Read the model definition and answer for the solid it produces. Units are mm, in the model's axes. A direction names the side the tool comes from. Give positions to 0.01 mm unless a question says otherwise; leave off trailing zeros. Write each loop counter-clockwise with the first axis right and the second up, starting at its lowest first coordinate (ties: lowest second). Pieces come first, ordered by that corner, then holes. Notation, with made-up numbers: (35.25, 58.5) -> (57.25, 58.5) arc R18 cw to (57.25, 63.5) -> close; hole circle Ø1 at (-11, 17.25). An arc over 180 degrees is marked (long way). Answer as CSV lines item,"result". Start each with the question number.
1. The part is cut by section C-C, the plane y = -49. Determine the outline of the cut face in (x, z) (1 decimal), and give its area (3 significant figures).
2. Given pin 1 (1.4 mm diameter, centred on y = -80.5, z = -0.5, fed in from -X); pin 2 (3 mm diameter, centred on y = -49.5, z = -6.5, fed in from -X); pin 3 (2 mm diameter, centred on y = -49.5, z = 1, fed in from +X), each flat-ended and moving along its own axis, determine where each tip first touches the part or whether it passes through.
3. The part is cut by section B-B, the plane y = -60. Determine the outline of the cut face in (x, z).
4. Find the intervals of material crossed by line 1 (Y direction, x = -90.5, z = 5.5); line 2 (X direction, y = -78, z = -5.5); line 3 (X direction, y = -75, z = 3.25), in increasing order.
5. The part is cut by section A-A, the plane x = -37. Determine the outline of the cut face in (y, z), and give its area (3 significant figures).
6. The part is cut by section D-D, the plane x = -15. Determine the outline of the cut face in (y, z), and give its area (3 significant figures).
7. A tool of negligible diameter and unlimited length cuts with its end or side. For faces 1 (the flat face through (-102.743, -74, -3)), 2 (the cylindrical face through (-22.46, -91.86, -1.69)), 3 (the cylindrical face through (-7.404, -76.068, -2.685)), 4 (the cylindrical face through (-22.46, -47.07, -1.69)), from which of +Z, -Z, +X, -X, +Y, -Y can it reach the whole face along a straight path? Write none if from no direction.
8. For a pull along Y with two mould halves and no side action, classify faces 5 (the cylindrical face through (-112.375, -77.345, 0.151)), 6 (the flat face through (-109.22, -80, 0)), 7 (the flat face through (-20, -50.165, 0)), 8 (the cylindrical face through (-93.667, -47.074, 0.909)) as pulls with the +Y half, pulls with the -Y half, needs draft (parallel to the pull), parting line crosses it, or undercut.
from build123d import *

# Parameters (mm, degrees)
SKETCH002_W     = 82.55
SKETCH002_H     = 25.4
PAD001_DEPTH    = 19.05
SKETCH003_R     = 5.08
POCKET001_DEPTH = 114.301
SKETCH100_R     = 2.286
POCKET027_DEPTH = 6.223
SKETCH101_R     = 7.14375
POCKET028_DEPTH = 12.7
SKETCH118_R     = 2.8575
POCKET042_DEPTH = 6.096


with BuildPart() as part:
    # Sketch002 → Pad001 (new body)
    with BuildSketch(Plane.XY):
        Polygon((-57.15, 14.589816), (-57.15, -14.589816), (-46.339816, -25.4), (46.339816, -25.4), (57.15, -14.589816), (57.15, 14.589816), (46.339816, 25.4), (-46.339816, 25.4), align=None)
        Rectangle(SKETCH002_W, SKETCH002_H, mode=Mode.SUBTRACT)
    extrude(amount=PAD001_DEPTH)

    # Sketch003 (on Face1 of Pad001) → Pocket001 (cut, through all)
    with BuildSketch(Plane(origin=(-57.15, 0, 0), x_dir=(0, -1, 0), z_dir=(-1, 0, 0))):
        with Locations((0, 9.525)):
            Circle(SKETCH003_R)
    extrude(amount=-POCKET001_DEPTH, mode=Mode.SUBTRACT)

    # Sketch100 (on Face1 of Pocket001) → Pocket027 (cut)
    with BuildSketch(Plane(origin=(-57.15, 0, 0), x_dir=(0, -1, 0), z_dir=(-1, 0, 0))):
        with Locations((10.16, 9.525)):
            Circle(SKETCH100_R)
        with Locations((-10.16, 9.525)):
            Circle(SKETCH100_R)
    extrude(amount=-POCKET027_DEPTH, mode=Mode.SUBTRACT)

    # Sketch101 (on Face1 of Pocket027) → Pocket028 (cut)
    with BuildSketch(Plane(origin=(-57.15, 0, 0), x_dir=(0, -1, 0), z_dir=(-1, 0, 0))):
        with Locations((0, 9.525)):
            Circle(SKETCH101_R)
    pocket028 = extrude(amount=-POCKET028_DEPTH, mode=Mode.SUBTRACT)

    # Mirrored002: Pocket028 across YZ
    add(pocket028.mirror(Plane.YZ), mode=Mode.SUBTRACT)

    # Sketch118 (on Face10 of Mirrored002) → Pocket042 (cut)
    with BuildSketch(Plane.XZ.offset(25.4)):
        with Locations((0, 9.525)):
            Circle(SKETCH118_R)
        with Locations((38.1, 9.525)):
            Circle(SKETCH118_R)
        with Locations((-38.1, 9.525)):
            Circle(SKETCH118_R)
    pocket042 = extrude(amount=-POCKET042_DEPTH, mode=Mode.SUBTRACT)

    # Mirrored004: Pocket042 across XZ
    add(pocket042.mirror(Plane.XZ), mode=Mode.SUBTRACT)


with BuildPart() as part_1:
    # Body001 placement: moved
    add(part.part.moved(Location((-58.293, -69.469, -9.4742))))


solid = part_1.part
Results found:
1,outline,"(-109.6, -9.5) -> (-7, -9.5) -> (-7, 9.6) -> (-109.6, 9.6) -> close; hole circle Ø5.7 at (-96.4, 0.1); hole circle Ø5.7 at (-58.3, 0.1); hole circle Ø5.7 at (-20.2, 0.1)"
1,area,"1,880 mm²"
2,pin 1,"stops at x = -109.22"
2,pin 2,"stops at x = -111.56"
2,pin 3,"stops at x = -5.52"
3,outline,"(-115.44, -9.47) -> (-99.57, -9.47) -> (-99.57, 9.58) -> (-115.44, 9.58) -> (-115.44, 2.23) -> (-109.22, 2.23) -> (-109.22, -2.13) -> (-115.44, -2.13) -> close; (-17.02, -9.47) -> (-1.14, -9.47) -> (-1.14, 9.58) -> (-17.02, 9.58) -> close"
4,line 1,"y = -94.87 to -82.17, -56.77 to -44.07"
4,line 2,"x = -115.44 to -99.57, -17.02 to -1.14"
4,line 3,"x = -102.74 to -99.57, -17.02 to -13.84"
5,outline,"(-94.87, -9.47) -> (-82.17, -9.47) -> (-82.17, 9.58) -> (-94.87, 9.58) -> close; (-56.77, -9.47) -> (-44.07, -9.47) -> (-44.07, 9.58) -> (-56.77, 9.58) -> close"
5,area,"484 mm²"
6,outline,"(-94.87, -9.47) -> (-44.07, -9.47) -> (-44.07, 9.58) -> (-94.87, 9.58) -> close; hole circle Ø10.16 at (-69.47, 0.05)"
6,area,"887 mm²"
7,face 1,"-X"
7,face 2,"-Y"
7,face 3,"+X"
7,face 4,"+Y"
8,face 5,"undercut"
8,face 6,"undercut"
8,face 7,"pulls with the +Y half"
8,face 8,"needs draft"
